from build123d import *

# Parameters (mm, degrees)
SKETCH_3_R = 0.423054932


with BuildPart() as part:
    # Эскиз1 → Повернуть2 (revolve)
    with BuildSketch(Plane(origin=(0, 0, 0), x_dir=(1, 0, 0), z_dir=(0, 1, 0))):
        with BuildLine():
            Line((-1.749578385, 0.423054932), (-1.749578385, 0))
            Line((-1.749578385, 0), (1.749578385, 0))
            Line((1.749578385, 0), (1.749578385, 0.423054932))
            ThreePointArc((1.749578385, 0.423054932), (1.144753012, 1.389079027), (0.080960724, 1.798178345))
            Line((0.080960724, 1.798178345), (0, 1.645856706))
            Line((0, 1.645856706), (-0.075759465, 1.798404989))
            ThreePointArc((-0.075759465, 1.798404989), (-1.142742977, 1.390733076), (-1.749578385, 0.423054932))
        make_face()
    revolve(axis=Axis((-29.751182373, 0, 0), (1, 0, 0)))

    # По траектории1: sweep along a path in Эскиз2
    with BuildLine(Plane.XY) as sweep_1_path:
        Line((0, 0), (-8, 0))
        ThreePointArc((-8, 0), (-8.707106781, -0.292893219), (-9, -1))
        Line((-9, -1), (-9, -11.514871198))
    # Эскиз3 → По траектории1 (sweep)
    with BuildSketch(Plane.ZY.offset(1.749578385)):
        Circle(SKETCH_3_R)
    sweep_1 = sweep(path=sweep_1_path.line)

    # Зеркальное отражение1: По траектории1 across plane
    add(sweep_1.mirror(Plane(origin=(0, 0, 0), x_dir=(0, 0, 1), z_dir=(1, 0, 0))))


solid = part.part
Read the model definition and answer for the solid it produces. Units are mm, in the model's axes. A direction names the side the tool comes from. Coordinates: 2 decimals unless noted, no trailing zeros. Write each loop counter-clockwise with the first axis right and the second up, starting at its lowest first coordinate (ties: lowest second). Pieces come first, ordered by that corner, then holes. Notation, with made-up numbers: (48.25, 13) -> (71.25, 13) arc R29 ccw to (71.25, 52) -> close; hole circle Ø11 at (45.5, 48.5). An arc over 180 degrees is marked (long way). Return JSON: item names as keys, results as strings.
(1) Which of the six approach directions +Z, -Z, +X, -X, +Y, -Y give full straight-line access (tool end or side, diameter ignored) to faces 1 (the cylindrical face through (-4.9, 0.3, -0.3)), 2 (the cylindrical face through (-9.42, -6.33, -0.06)), 3 (the flat face through (9, -11.515, 0))?
Answers below:
{"face 1": "none", "face 2": "-Y", "face 3": "+Z, -Z, +X, -X, -Y"}
(2) Each of these flat-tipped pins is pushed along its axis until it touches: P1, Ø1.5, axis at x = -1.5, z = -1.5, coming from the +Y side; P2, Ø1.5, axis at x = -1.5, z = 0, coming from the -Y side. Where does it stop, or does it pass through?
Answers below:
{"P1": "y = 1.17", "P2": "y = -1.64"}
(3) The part is cut by section C-C on x = -6.5. Give the vertices of the cut face in (y, z).
Answers below:
{"outline": "circle Ø0.85 at (0, 0)"}
(4) The part is cut by section A-A on y = -6.75. Give the vertices of the cut face in (x, z), then the cut area to 3 significant figures.
Answers below:
{"outline": "circle Ø0.85 at (-9, 0); circle Ø0.85 at (9, 0)", "area": "1.12 mm^2"}
(5) The part is cut by section B-B on z = 0. Give the vertices of the cut face in (x, y).
Answers below:
{"outline": "(-9.42, -11.51) -> (-8.58, -11.51) -> (-8.58, -1) arc R0.58 cw to (-8, -0.42) -> (-1.75, -0.42) arc R1.8 ccw to (-0.08, -1.8) -> (0, -1.65) -> (0.08, -1.8) arc R1.8 ccw to (1.75, -0.42) -> (8, -0.42) arc R0.58 cw to (8.58, -1) -> (8.58, -11.51) -> (9.42, -11.51) -> (9.42, -1) arc R1.42 ccw to (8, 0.42) -> (1.75, 0.42) arc R1.8 ccw to (0.08, 1.8) -> (0, 1.65) -> (-0.08, 1.8) arc R1.8 ccw to (-1.75, 0.42) -> (-8, 0.42) arc R1.42 ccw to (-9.42, -1) -> close"}
(6) Consider line 1 along X through (y, z) = (-6.5, -0.05); line 2 along X through (y, z) = (-0.5, 0.3); line 3 along Y through (x, z) = (-8, 0). Determine where each line is inside the solid, lowest interval first. Write a range as from..to.
Answers below:
{"line 1": "-9.42..-8.58, 8.58..9.42", "line 2": "-9.2..-8.49, -1.7..1.7, 8.49..9.2", "line 3": "-0.42..0.42"}
(7) The part is cut by section D-D on y = -1.5. State how many separate pieces and enclosed holes the cut face has, then the cut area to 3 significant figures.
Answers below:
{"separate pieces": "3", "enclosed holes": "0", "area": "4.19 mm^2"}
